```python
from build123d import *

# Parameters (mm, degrees)
F2_W     = 3.175
F2_H     = 8.4529162467
F3_DEPTH = 46.228
F5_D     = 3.4544
F5_DEPTH = 15.08125
F5_TIP   = 1.0378064612


with BuildPart() as f1:
    # F0 (on Front) → F1 (revolve)
    with BuildSketch(Plane.XZ):
        Polygon((0, 6.35), (0, 0), (166.624, 0), (166.624, 4.7625), (153.924, 4.7625), (153.924, 38.862), (50.8, 38.862), (50.8, 17.4498), (46.228, 17.4498), (46.228, 6.35), align=None)
    revolve(axis=Axis((76.633890767, 0, 0), (1, 0, 0)))

    # F2 (on face) → F3 (cut, through all)
    with BuildSketch(Plane(origin=(0, 0, 0), x_dir=(0, -1, 0), z_dir=(-1, 0, 0))):
        with Locations((0, 7.4014581233)):
            Rectangle(F2_W, F2_H)
    extrude(amount=-F3_DEPTH, mode=Mode.SUBTRACT)

    # F5
    with Locations(Plane(origin=(50.8, 0, 0), x_dir=(0, -1, 0), z_dir=(-1, 0, 0))):
        with Locations((-25, 0), (0, -25), (25, 0), (0, 25)):
            Hole(F5_D / 2, depth=F5_DEPTH)
            with Locations((0, 0, -(F5_DEPTH + F5_TIP / 2))):  # 118° drill point
                Cone(0, F5_D / 2, F5_TIP, mode=Mode.SUBTRACT)


solid = f1.part
```
Build history of the part. All positions in model axes, mm. A direction names the side the tool comes from. Round coordinates to 2 decimals unless told otherwise and drop trailing zeros. Loops run counter-clockwise (first coordinate to the right, second up) from the corner with the lowest first, then second, coordinate; pieces in that order, holes last. Notation, with made-up numbers: M -19,-28.75 L -14,-28.75 A16 ccw -14,1.25 Z; hole C 15.25,18.25 d5. An arc over 180 degrees is marked long. Answer as CSV lines item,"result".
1. 3-axis set-ups, long thin cutter, end or side, ignore diameter. For faces 5 (the cylindrical face through (160.19, 2.9, -3.78)), 6 (the cylindrical face through (101.64, 37.94, -8.42)), 7 (the flat face through (0, 0, 0)), 8 (the flat face through (23, 0, 3.175)), 9 (the flat face through (50.8, 8, 17)): which of +Z, -Z, +X, -X, +Y, -Y reach the whole face in a straight line?
Resolved:
face 5,"+X"
face 6,"+X, -X"
face 7,"+Z, -Z, -X, +Y, -Y"
face 8,"+Z, -X"
face 9,"-X"
2. Cut at C-C on x = 143. Write the cut outline in (y, z).
Resolved:
outline,"C 0,0 d77.72"
3. Cut at A-A on z = -15. Write the cut outline in (x, y), then the cut area to 3 significant figures.
Resolved:
outline,"M 46.23,-8.92 L 50.8,-8.92 L 50.8,-35.85 L 153.92,-35.85 L 153.92,35.85 L 50.8,35.85 L 50.8,8.92 L 46.23,8.92 Z"
area,"7,480 mm²"
4. Wall check: probe 1 along Z at (x, y) = (58, 0); probe 2 along X at (y, z) = (22.5, 6.5). Give the ranges that are in metal, low to high. Write a range as [from, to].
Resolved:
probe 1,"z = [-38.86, -26.73], [-23.27, 23.27], [26.73, 38.86]"
probe 2,"x = [50.8, 153.92]"
5. Cut at D-D on y = 32.5. Write the cut outline in (x, z), then the cut area to 3 significant figures.
Resolved:
outline,"M 50.8,-21.31 L 153.92,-21.31 L 153.92,21.31 L 50.8,21.31 Z"
area,"4,390 mm²"
6. Cut at B-B on y = 13. Write the cut outline in (x, z).
Resolved:
outline,"M 46.23,-11.64 L 50.8,-11.64 L 50.8,-36.62 L 153.92,-36.62 L 153.92,36.62 L 50.8,36.62 L 50.8,11.64 L 46.23,11.64 Z"
7. Flat gauge pins, fed straight in: P1, Ø4, axis at x = 109, y = -23, coming from the -Z side; P2, Ø1, axis at x = 28, y = 0.5, coming from the +Z side (3 decimals); P3, Ø4.5, axis at y = 0, z = 25, coming from the +X side. Where does each tip first touch, or does it go through?
Resolved:
P1,"stops at z = -32.7"
P2,"stops at z = 3.175"
P3,"stops at x = 153.92"
8. Two-plate mould, pull along Z, no slides. Class faces 1 (the cylindrical face through (22.79, -0.257, -6.345)), 2 (the cylindrical face through (58.446, -0.225, 26.713)), 3 (the flat face through (46.228, 0, 4)), 4 (the conical face through (66.74, 25.22, 0.2)): released by +Z, released by -Z, zero draft, split by the parting line, or undercut.
Resolved:
face 1,"split by the parting line"
face 2,"undercut"
face 3,"zero draft"
face 4,"undercut"
